Can you work these out from the model? Positions are in its coordinate system, mm. A direction names the side the tool comes from. Round coordinates to 2 decimals unless told otherwise and drop trailing zeros. Write each loop counter-clockwise with the first axis right and the second up, starting at its lowest first coordinate (ties: lowest second). Pieces come first, ordered by that corner, then holes. Notation, with made-up numbers: M 10,76.5 L 59,76.5 A14 ccw 59,101.5 Z; hole C 57,75.25 d2. An arc over 180 degrees is marked long. Answer in a Markdown table with one row per item. Add a question column.
(1) Suppose I cut it at B-B, the plane y = 2.5. Count the separate pieces of the cut face and the enclosed holes in it, then the cut area to 3 significant figures.
(2) If I drill on probe 1 along X at (y, z) = (7.75, 0) (3 decimals); probe 2 along Z at (x, y) = (-24.5, 1); probe 3 along X at (y, z) = (1, 1), over which ranges is the centre line in solid material (lowest first)?
(3) If we mould it in two halves opening along X, with no side actions, what happens to faces 1 (the face through (0, 11, 0)), 2 (the face through (0, 10, 0))? For each: released by +X, released by -X, zero draft, split by the parting line, or undercut.
(4) For faces 3 (the face through (-28, 10, 0)), 4 (the face through (25, 0, 0)), which set-ups out of +Z, -Z, +X, -X, +Y, -Y let a thin tool reach every point of the face, with its end or its side?
(5) Suppose I cut it at A-A, the plane z = 0. Write out the boundary of the cut face in (x, y) (3 decimals), then the cut area to 3 significant figures.
(6) I'm going to push flat-ended pins straight in: pin 1 (10 mm diameter, centred on x = 1, z = 5, fed in from -Y); pin 2 (0.8 mm diameter, centred on y = 10.5, z = 12.5, fed in from -X); pin 3 (0.8 mm diameter, centred on y = 10.5, z = 12, fed in from +X). Where does each tip first touch, or does it pass through?
from build123d import *

# Parameters (mm, degrees)
SKIZZE1_R                       = 30.405
SKIZZE1_R_2                     = 28.405
AUFSATZ_LINEAR_AUSTRAGEN1_DEPTH = 10
SKIZZE2_R                       = 30.405
AUFSATZ_LINEAR_AUSTRAGEN2_DEPTH = 1
AUFSATZ_LINEAR_START            = 10
AUFSATZ_LINEAR_AUSTRAGEN3_DEPTH = 10
SKIZZE5_R                       = 1.5
SCHNITT_LINEAR_AUSTRAGEN2_DEPTH = 10
SKIZZE6_W                       = 7.2
SKIZZE6_H                       = 10
SCHNITT_LINEAR_AUSTRAGEN3_DEPTH = 10
KREISMUSTER1_COUNT              = 2
KREISMUSTER1_ANGLE              = 90
FASE1_SIZE                      = 1
VERRUNDUNG1_R                   = 2
VERRUNDUNG2_R                   = 1
FASE2_SIZE                      = 1


with BuildPart() as part:
    # Skizze1 → Aufsatz-Linear austragen1 (new body)
    with BuildSketch(Plane(origin=(0, 0, 0), x_dir=(1, 0, 0), z_dir=(0, 1, 0))):
        with Locations(Location((0, 0, 0), (0, 0, 270))):
            Circle(SKIZZE1_R)
        with Locations(Location((0, 0, 0), (0, 0, 270))):
            Circle(SKIZZE1_R_2, mode=Mode.SUBTRACT)
    extrude(amount=AUFSATZ_LINEAR_AUSTRAGEN1_DEPTH)

    # Skizze2 → Aufsatz-Linear austragen2 (add)
    with BuildSketch(Plane(origin=(0, 10, 0), x_dir=(1, 0, 0), z_dir=(0, 1, 0))):
        with Locations(Location((0, 0, 0), (0, 0, 270))):
            Circle(SKIZZE2_R)
    extrude(amount=AUFSATZ_LINEAR_AUSTRAGEN2_DEPTH)

    # Skizze4 → Aufsatz-Linear austragen3 (add)
    with BuildSketch(Plane.XZ.offset(-10).offset(AUFSATZ_LINEAR_START)):
        with BuildLine():
            ThreePointArc((-28.07385528, -4.324658914), (-23.255, 0), (-28.07385528, 4.324658914))
            ThreePointArc((-28.07385528, 4.324658914), (-28.405, 0), (-28.07385528, -4.324658914))
        make_face()
        with BuildLine():
            ThreePointArc((28.405, 0), (28.322092827, 2.168659237), (28.07385528, 4.324658914))
            ThreePointArc((28.07385528, 4.324658914), (23.255, 0), (28.07385528, -4.324658914))
            ThreePointArc((28.07385528, -4.324658914), (28.322092827, -2.168659237), (28.405, 0))
        make_face()
    aufsatz_linear_austragen3 = extrude(amount=-AUFSATZ_LINEAR_AUSTRAGEN3_DEPTH)

    # Skizze5 → Schnitt-Linear austragen2 (cut)
    with BuildSketch(Plane.XZ):
        with Locations(Location((-27.605, 0, 0), (0, 0, 270))):
            Circle(SKIZZE5_R)
        with BuildLine():
            ThreePointArc((29.105, 0), (27.605, 1.5), (26.105, 0))
            Line((26.105, 0), (29.105, 0))
        make_face()
        with BuildLine():
            Line((29.105, 0), (26.105, 0))
            ThreePointArc((26.105, 0), (27.605, -1.5), (29.105, 0))
        make_face()
    schnitt_linear_austragen2 = extrude(amount=-SCHNITT_LINEAR_AUSTRAGEN2_DEPTH, mode=Mode.SUBTRACT)

    # Skizze6 → Schnitt-Linear austragen3 (cut)
    with BuildSketch(Plane(origin=(0, 11, 0), x_dir=(1, 0, 0), z_dir=(0, 1, 0))):
        with Locations((3.69194255, -10.988)):
            Rectangle(SKIZZE6_W, SKIZZE6_H)
    extrude(amount=-SCHNITT_LINEAR_AUSTRAGEN3_DEPTH, mode=Mode.SUBTRACT)

    # Kreismuster1: Aufsatz-Linear austragen3, Schnitt-Linear austragen2 ×2 about axis
    kreismuster1_axis = Axis((0, 0, 0), (0, 1, 0))
    add([aufsatz_linear_austragen3.rotate(kreismuster1_axis, i * KREISMUSTER1_ANGLE / (KREISMUSTER1_COUNT - 1)) for i in range(1, KREISMUSTER1_COUNT)])
    add([schnitt_linear_austragen2.rotate(kreismuster1_axis, i * KREISMUSTER1_ANGLE / (KREISMUSTER1_COUNT - 1)) for i in range(1, KREISMUSTER1_COUNT)], mode=Mode.SUBTRACT)

    # Fase1
    fase1_edges = [part.edges().sort_by_distance(p)[0] for p in [
        (0, 11, -30.405),
    ]]
    chamfer(fase1_edges, length=FASE1_SIZE)

    # Verrundung1
    verrundung1_edges = [part.edges().sort_by_distance(p)[0] for p in [
        (-28.07385528, 5, 4.324658914),
        (-28.07385528, 5, -4.324658914),
        (28.07385528, 5, 4.324658914),
        (28.07385528, 5, -4.324658914),
        (4.324658914, 5, 28.07385528),
        (-4.324658914, 5, 28.07385528),
        (4.324658914, 5, -28.07385528),
        (-4.324658914, 5, -28.07385528),
    ]]
    fillet(verrundung1_edges, radius=VERRUNDUNG1_R)

    # Verrundung2
    verrundung2_edges = [part.edges().sort_by_distance(p)[0] for p in [
        (7.29194255, 10.5, 5.988),
        (7.29194255, 10.5, 15.988),
        (0.09194255, 10.5, 15.988),
        (0.09194255, 10.5, 5.988),
    ]]
    fillet(verrundung2_edges, radius=VERRUNDUNG2_R)

    # Fase2
    fase2_edges = [part.edges().sort_by_distance(p)[0] for p in [
        (-20.08536812, 10, -20.08536812),
        (0, 10, -23.255),
        (20.08536812, 10, -20.08536812),
        (23.255, 10, 0),
        (20.08536812, 10, 20.08536812),
        (0, 10, 23.255),
        (-20.08536812, 10, 20.08536812),
        (-23.255, 10, 0),
        (-5.068546935, 10, 27.438977106),
        (5.068546935, 10, 27.438977106),
        (-27.438977106, 10, -5.068546935),
        (-27.438977106, 10, 5.068546935),
        (27.438977106, 10, 5.068546935),
        (27.438977106, 10, -5.068546935),
        (5.068546935, 10, -27.438977106),
        (-5.068546935, 10, -27.438977106),
    ]]
    chamfer(fase2_edges, length=FASE2_SIZE)


solid = part.part
Calculated:
| question | item | result |
|---|---|---|
| 1 | separate pieces | 1 |
| 1 | enclosed holes | 5 |
| 1 | area | 491 mm² |
| 2 | probe 1 | -30.405 to -29.105, -26.105 to -23.255, 23.255 to 26.105, 29.105 to 30.405 |
| 2 | probe 2 | -18.01 to -14.37, -3.05 to 3.05, 14.37 to 18.01 |
| 2 | probe 3 | -30.39 to -28.72, -26.49 to -23.37, 23.37 to 26.49, 28.72 to 30.39 |
| 3 | face 1 | zero draft |
| 3 | face 2 | undercut |
| 4 | face 3 | -Y |
| 4 | face 4 | +Z, -Z, +X, -X, -Y |
| 5 | outline | M -30.405,0 L -29.105,0 L -29.105,10 L -26.105,10 L -26.105,0 L -23.255,0 L -23.255,9 L -22.255,10 L 22.255,10 L 23.255,9 L 23.255,0 L 26.105,0 L 26.105,10 L 29.105,10 L 29.105,0 L 30.405,0 L 30.405,10 L 29.405,11 L -29.405,11 L -30.405,10 Z |
| 5 | area | 144 mm² |
| 6 | pin 1 | y = 10 |
| 6 | pin 2 | x = -27.64 |
| 6 | pin 3 | x = 27.86 |
